Part model, mm, in its own coordinate system. A direction names the side the tool comes from. Round coordinates to 2 decimals unless told otherwise and drop trailing zeros. Order: outer loops, then holes, each group sorted by start corner. A loop starts at its lowest first (then second) coordinate and runs counter-clockwise, first axis right, second up. Notation, with made-up numbers: M 46,-38 L 65,-38 A16 cw 65,-14 Z; hole C 22.5,-11.5 d5. An arc over 180 degrees is marked long. Write each question's results on one line, items separated by ' | '. Start each with the question number.
1. Band-saw the part on A-A, the plane z = 16.75. List the corners of the cut face in (x, y), then the cut area to 3 significant figures.
2. Band-saw the part on B-B, the plane x = 35. List the corners of the cut face in (y, z), then the cut area to 3 significant figures.
3. Probe L1, parallel to Z at x = 155, y = 166; L2, parallel to Y at x = 123, z = 9; L3, parallel to X at y = 129.5, z = 15.5. List the from-to ranges inside material, lowest first. Write a range as [from, to].
4. Which spindle directions (+Z, -Z, +X, -X, +Y, -Y) get a long thin tool onto all of the face, cutting with end or side? Do faces 4 (the face through (97, 108, 1.588)), 5 (the face through (87.66, 123.58, 12.52)). Say none if no direction does.
5. Band-saw the part on C-C, the plane y = 89. List the corners of the cut face in (x, z).
6. Band-saw the part on D-D, the plane y = 28. List the corners of the cut face in (x, z).
7. Drop flat-ended pins along their axis: pin 1 Ø6 at (y, z) = (93.5, 16) entering from +X; pin 2 Ø5 at (y, z) = (181.5, 9) entering from +X; pin 3 Ø4 at (x, z) = (177, 16.5) entering from -Y. Give the stop position or say it passes through.
8. Two-plate mould, pull along X, no slides. Class faces 1 (the face through (196, 213.721, 1)), 2 (the face through (108, 108, 13)), 3 (the face through (88.762, 122.438, 12.544)): +X half, -X half, draft (parallel to the pull), parting line (faces both ways), or undercut.
Autodesk Inventor part; units mm, degrees
ref_plane "YZ Plane" through (0, 0, 0) normal (1, 0, 0) x (0, 1, 0)
ref_plane "XZ Plane" through (0, 0, 0) normal (0, 1, 0) x (-1, 0, 0)
ref_plane "XY Plane" through (0, 0, 0) normal (0, 0, 1) x (1, 0, 0)
sketch "Sketch1" plane through (0, 0, 0) normal (0, 0, 1) x (1, 0, 0)
  line L0 (0, 0) -> (0, 35.921)
  line L1 (0, 35.921) -> (177.8, 213.721)
  line L2 (177.8, 213.721) -> (213.721, 213.721)
  line L3 (213.721, 213.721) -> (0, 0)
  dimension "d0" = 25.4
  dimension "d2" = 177.8
  dimension "d3" = 177.8
extrude "Extrusion1" add sketch "Sketch1" along normal blind 25.4
shell "Shell1" thickness 1.5875 removed faces 2 at (0, 11.9737, 8.4667) at (189.7737, 213.721, 16.9333)
properties part number "Frame_VerticalFrontAngle" material "Aluminum-6061"
Solution:
1) outline: M 0,0 L 213.72,213.72 L 211.48,213.72 L 0,2.25 Z; M 0,33.68 L 180.05,213.72 L 177.8,213.72 L 0,35.92 Z | area: 879 mm^2
2) outline: M 35,0 L 70.92,0 L 70.92,25.4 L 35,25.4 Z; hole M 37.25,1.59 L 68.68,1.59 L 68.68,23.81 L 37.25,23.81 Z | area: 214 mm^2
3) L1: [0, 1.59], [23.81, 25.4] | L2: [123, 125.25], [156.68, 158.92] | L3: [93.58, 95.82], [127.25, 129.5]
4) face 4: none | face 5: +Z, -Z, -X, +Y
5) outline: M 53.08,0 L 89,0 L 89,25.4 L 53.08,25.4 Z; hole M 55.32,1.59 L 86.75,1.59 L 86.75,23.81 L 55.32,23.81 Z
6) outline: M 0,0 L 28,0 L 28,25.4 L 0,25.4 L 0,23.81 L 25.75,23.81 L 25.75,1.59 L 0,1.59 Z
7) pin 1: x = 96.5 | pin 2: x = 184 | pin 3: y = 175
8) face 1: draft | face 2: +X half | face 3: undercut
